Part print with two shaded views. Sizes in mm from the minimum x, y, z corner. Round coordinates to 2 decimals unless told otherwise and drop trailing zeros. Write each loop counter-clockwise with the first axis right and the second up, starting at its lowest first coordinate (ties: lowest second). Pieces come first, ordered by that corner, then holes. Notation, with made-up numbers: (87.5, 82.25) -> (106.5, 82.25) arc R19 ccw to (106.5, 93.25) -> close; hole circle Ø4 at (73.5, -19). An arc over 180 degrees is marked (long way). Return JSON: item names as keys, results as strings.
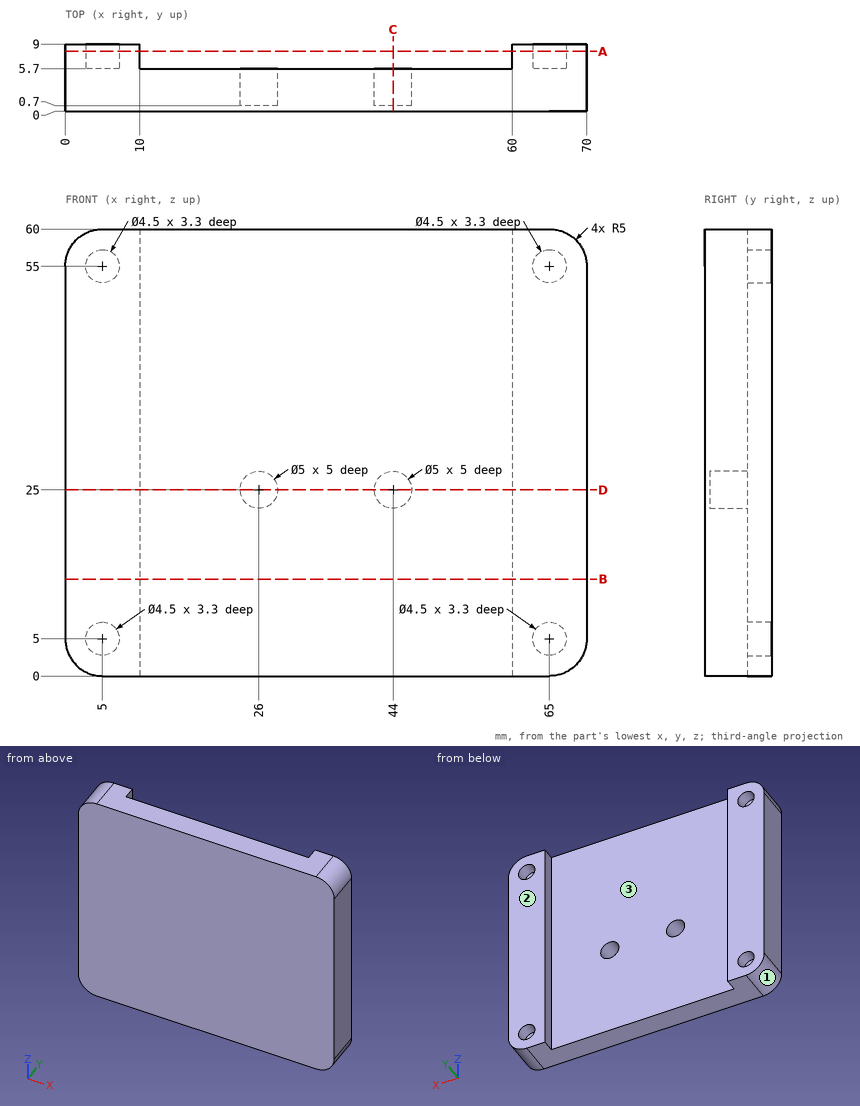
Q1. Saw through at C-C on x = 44. List the corners of the cut face in (y, z), then the cut area to 3 significant figures.
Verdict:
{"outline": "(0, 0) -> (5.7, 0) -> (5.7, 22.5) -> (0.7, 22.5) -> (0.7, 27.5) -> (5.7, 27.5) -> (5.7, 60) -> (0, 60) -> close", "area": "317 mm²"}
Q2. Saw through at D-D on z = 25. List the corners of the cut face in (x, y), then the cut area to 3 significant figures.
Verdict:
{"outline": "(0, 0) -> (70, 0) -> (70, 9) -> (60, 9) -> (60, 5.7) -> (46.5, 5.7) -> (46.5, 0.7) -> (41.5, 0.7) -> (41.5, 5.7) -> (28.5, 5.7) -> (28.5, 0.7) -> (23.5, 0.7) -> (23.5, 5.7) -> (10, 5.7) -> (10, 9) -> (0, 9) -> close", "area": "415 mm²"}
Q3. Two-plate mould, pull along X, no slides. Class the marked faces 1, 2 and 3: +X half, -X half, draft (parallel to the pull), parting line (faces both ways), or undercut.
Verdict:
{"face 1": "-X half", "face 2": "draft", "face 3": "undercut"}
Q4. Pin check, flat tips, straight feed: pin 1 Ø6.5 at (x, z) = (26, 25) entering from +Y; pin 2 Ø2.5 at (x, z) = (44, 25) entering from +Y. Stop position of each tip, or through.
Verdict:
{"pin 1": "stops at y = 5.7", "pin 2": "stops at y = 0.7"}
Q5. Saw through at B-B on z = 13. List the corners of the cut face in (x, y), then the cut area to 3 significant figures.
Verdict:
{"outline": "(0, 0) -> (70, 0) -> (70, 9) -> (60, 9) -> (60, 5.7) -> (10, 5.7) -> (10, 9) -> (0, 9) -> close", "area": "465 mm²"}
Q6. Saw through at A-A on y = 8. List the corners of the cut face in (x, z).
Verdict:
{"outline": "(0, 5) arc R5 ccw to (5, 0) -> (10, 0) -> (10, 60) -> (5, 60) arc R5 ccw to (0, 55) -> close; (60, 0) -> (65, 0) arc R5 ccw to (70, 5) -> (70, 55) arc R5 ccw to (65, 60) -> (60, 60) -> close; hole circle Ø4.5 at (5, 5); hole circle Ø4.5 at (5, 55); hole circle Ø4.5 at (65, 5); hole circle Ø4.5 at (65, 55)"}
Q7. Wall check: L1, parallel to X at y = 2.6, z = 25; L2, parallel to X at y = 7.95, z = 55; L3, parallel to Z at x = 65, y = 7.45. Give the ranges that are in metal, low to high.
Verdict:
{"L1": "x = 0 to 23.5, 28.5 to 41.5, 46.5 to 70", "L2": "x = 0 to 2.75, 7.25 to 10, 60 to 62.75, 67.25 to 70", "L3": "z = 0 to 2.75, 7.25 to 52.75, 57.25 to 60"}
